Verification items for this drawing (mm, ordinates from the low corner). A direction names the side the tool comes from. Round coordinates to 2 decimals unless told otherwise and drop trailing zeros. Order: outer loops, then holes, each group sorted by start corner. A loop starts at its lowest first (then second) coordinate and runs counter-clockwise, first axis right, second up. Notation, with made-up numbers: (-35.5, 41) -> (-12.5, 41) arc R31 ccw to (-12.5, 74) -> close; hole circle Ø7 at (-23, 69.25). An arc over 180 degrees is marked (long way). Return JSON: item names as keys, results as strings. Group by question number.
Item 1: Sectioned sample at D-D on x = 17. Record the cut outline in (y, z), plus the area to 3 significant figures.
Item 2: Sectioned sample at C-C on x = 29. Record the cut outline in (y, z).
Item 3: Scan lines: probe 1 along Y at (x, z) = (5, 17.75); probe 2 along Z at (x, y) = (17, 3.5); probe 3 along Z at (x, y) = (32.5, 8.25). Record each from-to range of solid material in increasing order. Write a range as from..to.
Item 4: Sectioned sample at A-A on y = 6. Record the cut outline in (x, z) (1 decimal), plus the area to 3 significant figures.
Item 5: Access from +Z, -Z, +X, -X, +Y, -Y to the whole of each face (thin tool, end or side, straight path). Record for the marked faces 5, 6 and 7.
Item 6: Depth check by flat-ended pin: pin 1 Ø5 at (x, y) = (5, 6) entering from -Z; pin 2 Ø3 at (y, z) = (14, 11.5) entering from -X; pin 3 Ø12 at (y, z) = (7, 7.5) entering from +X. Enter the tip coordinate at first touch or a pass-through.
Item 7: Sectioned sample at B-B on z = 11. Record the cut outline in (x, y), plus the area to 3 significant figures.
Item 8: Draft check along Z on the marked faces 1, 2, 3 and 4. Enter one of: pulls with the +Z half, pulls with the -Z half, needs draft (parallel to the pull), parting line crosses it, or undercut.
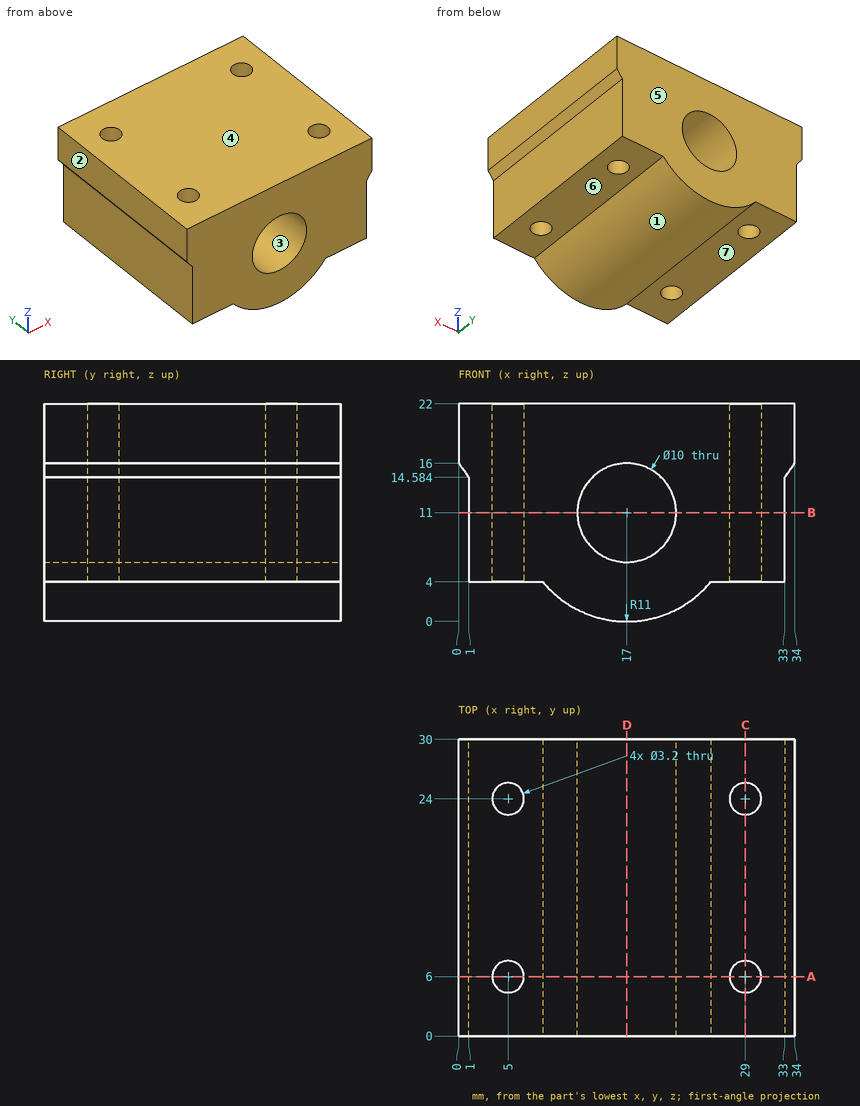
Recorded:
{
 "1": {"outline": "(0, 0) -> (30, 0) -> (30, 6) -> (0, 6) -> close; (0, 16) -> (30, 16) -> (30, 22) -> (0, 22) -> close", "area": "360 mm²"},
 "2": {"outline": "(0, 4) -> (4.4, 4) -> (4.4, 22) -> (0, 22) -> close; (7.6, 4) -> (22.4, 4) -> (22.4, 22) -> (7.6, 22) -> close; (25.6, 4) -> (30, 4) -> (30, 22) -> (25.6, 22) -> close"},
 "3": {"probe 1": "0..4.4, 7.6..22.4, 25.6..30", "probe 2": "0..6, 16..22", "probe 3": "4..22"},
 "4": {"outline": "(0, 16) -> (1, 14.6) -> (1, 4) -> (3.4, 4) -> (3.4, 22) -> (0, 22) -> close; (6.6, 4) -> (8.5, 4) arc R11 ccw to (25.5, 4) -> (27.4, 4) -> (27.4, 22) -> (6.6, 22) -> close; (30.6, 4) -> (33, 4) -> (33, 14.6) -> (34, 16) -> (34, 22) -> (30.6, 22) -> close; hole circle Ø10 at (17, 11)", "area": "443 mm²"},
 "5": {"face 5": "+Z, -Z, +X, -X, +Y", "face 6": "-Z, +X, +Y, -Y", "face 7": "-Z, -X, +Y, -Y"},
 "6": {"pin 1": "z = 4", "pin 2": "x = 1", "pin 3": "x = 33"},
 "7": {"outline": "(1, 0) -> (12, 0) -> (12, 30) -> (1, 30) -> close; (22, 0) -> (33, 0) -> (33, 30) -> (22, 30) -> close; hole circle Ø3.2 at (5, 6); hole circle Ø3.2 at (5, 24); hole circle Ø3.2 at (29, 6); hole circle Ø3.2 at (29, 24)", "area": "628 mm²"},
 "8": {"face 1": "pulls with the -Z half", "face 2": "needs draft", "face 3": "undercut", "face 4": "pulls with the +Z half"}
}
